Design review of the part shown in the three views and the two pictorial views. Dimensions are in mm from the part's minimum x, y and z. A direction names the side the tool comes from. Give positions to 0.01 mm unless a question says otherwise; leave off trailing zeros. Order: outer loops, then holes, each group sorted by start corner. A loop starts at its lowest first (then second) coordinate and runs counter-clockwise, first axis right, second up.
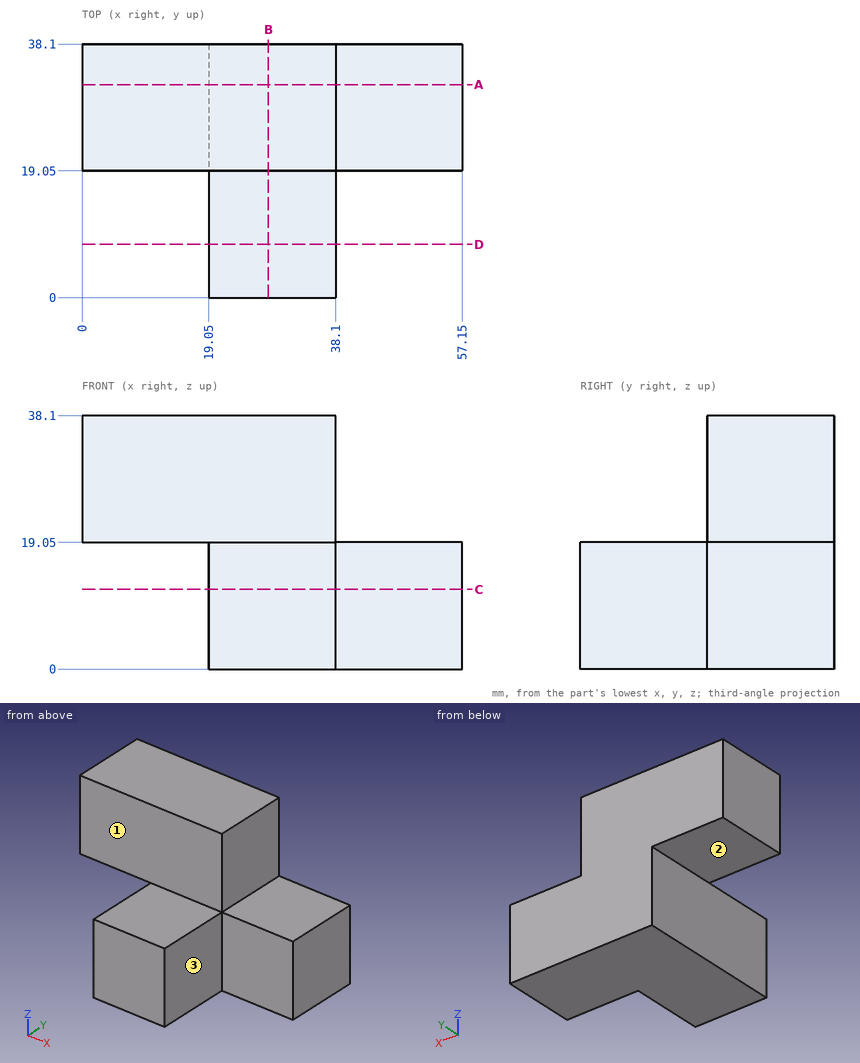
Item 1: Take a section at C-C (z = 12). Give the boundary of the cut face in (x, y).
Values found:
outline: (19.05, 0) - (38.1, 0) - (38.1, 19.05) - (57.15, 19.05) - (57.15, 38.1) - (19.05, 38.1) - close
Item 2: Clearance check with flat-ended pins moving along their axes: pin 1 Ø5.5 at (y, z) = (27, 33) entering from +X; pin 2 Ø15 at (x, y) = (7, 28) entering from -Z; pin 3 Ø1 at (x, z) = (22.5, 21) entering from -Y. State where each tip first meets the part, or that it passes through.
Values found:
pin 1: stops at x = 38.1
pin 2: stops at z = 19.05
pin 3: stops at y = 19.05
Item 3: For the marked faces 1, 2 and 3, list the 3-axis set-ups (+Z, -Z, +X, -X, +Y, -Y) from which the entire face can be reached by the end or side of a thin tool; tool diameter is ignored.
Values found:
face 1: +Z, +X, -X, -Y
face 2: -Z, -X, +Y, -Y
face 3: +Z, -Z, +X, -Y
Item 4: Take a section at B-B (x = 28). Give the boundary of the cut face in (y, z), and give its area (3 significant figures).
Values found:
outline: (0, 0) - (38.1, 0) - (38.1, 38.1) - (19.05, 38.1) - (19.05, 19.05) - (0, 19.05) - close
area: 1,090 mm2
Item 5: Take a section at D-D (y = 8). Give the boundary of the cut face in (x, z).
Values found:
outline: (19.05, 0) - (38.1, 0) - (38.1, 19.05) - (19.05, 19.05) - close
Item 6: For line 1 (Y direction, x = 49.5, z = 15.5); line 2 (X direction, y = 24.5, z = 17.5), list the stretches that pass through material, from the lowest coordinate up.
Values found:
line 1: y = 19.05 to 38.1
line 2: x = 19.05 to 57.15
Item 7: Take a section at A-A (y = 32). Give the boundary of the cut face in (x, z).
Values found:
outline: (0, 19.05) - (19.05, 19.05) - (19.05, 0) - (57.15, 0) - (57.15, 19.05) - (38.1, 19.05) - (38.1, 38.1) - (0, 38.1) - close
